from build123d import *

# Parameters (mm, degrees)
EXTRUDE1_DEPTH      = 8
EXTRUDE1_DEPTH_BACK = 8
SKETCH2_W           = 6.5
SKETCH2_H           = 12.5625
SKETCH3_W           = 94
SKETCH3_H           = 94
EXTRUDE2_DEPTH      = 31
SKETCH4_W           = 94
SKETCH4_H           = 47
EXTRUDE3_DEPTH      = 14
EXTRUDE3_DEPTH_BACK = 14
EXTRUDE4_DEPTH      = 2.06
EXTRUDE4_DEPTH_BACK = 2.06


with BuildPart() as part:
    # Sketch1 → Extrude1 (new body, two sides)
    with BuildSketch(Plane.XY) as extrude1_sk:
        with BuildLine():
            Line((-6.51, 14.5), (6.49, 14.5))
            ThreePointArc((6.49, 14.5), (10.317505243, 16.512584876), (14.256035557, 18.29815852))
            ThreePointArc((14.256035557, 18.29815852), (15.968337207, 18.822804929), (17.75042382, 19))
            Line((17.75042382, 19), (23.046668584, 19))
            ThreePointArc((23.046668584, 19), (24.290541726, 19.085889358), (25.51080482, 19.341927159))
            Line((25.51080482, 19.341927159), (35.534460964, 22.178335945))
            ThreePointArc((35.534460964, 22.178335945), (38.480369536, 24.039582758), (39.938965898, 27.204249197))
            Line((39.938965898, 27.204249197), (40.03902701, 27.893511518))
            ThreePointArc((40.03902701, 27.893511518), (39.384905735, 30.021406047), (37.324018346, 30.863161913))
            ThreePointArc((37.324018346, 30.863161913), (16.196447137, 28.065543342), (-4.25177913, 22.059631473))
            ThreePointArc((-4.25177913, 22.059631473), (-5.890644629, 20.775261015), (-6.51, 18.787325774))
            Line((-6.51, 18.787325774), (-6.51, 14.5))
        make_face()
    extrude(amount=EXTRUDE1_DEPTH)
    extrude(extrude1_sk.sketch, amount=-EXTRUDE1_DEPTH_BACK)

    # Sketch2 → Revolve1 (revolve)
    with BuildSketch(Plane.XY):
        with Locations((-3.26, 10.28125)):
            Rectangle(SKETCH2_W, SKETCH2_H)
    revolve(axis=Axis((-0.01, 16.5625, 0), (0, -1, 0)))

    # Sketch3 → Extrude2 (cut)
    with BuildSketch(Plane(origin=(0, 31, 0), x_dir=(-1, 0, 0), z_dir=(0, 1, 0))):
        with Locations((-7, -7)):
            Rectangle(SKETCH3_W, SKETCH3_H)
        with BuildLine():
            Line((-20.791020756, 4.081513031), (-36.5, 3.5))
            ThreePointArc((-36.5, 3.5), (-40, 0), (-36.5, -3.5))
            Line((-36.5, -3.5), (-20.791020756, -4.081513031))
            ThreePointArc((-20.791020756, -4.081513031), (-20.282143055, -4.074432197), (-19.7766212, -4.015658847))
            ThreePointArc((-19.7766212, -4.015658847), (-11.97399514, -3.733401658), (-4.362785826, -5.474130053))
            ThreePointArc((-4.362785826, -5.474130053), (7, 0), (-4.362785826, 5.474130053))
            ThreePointArc((-4.362785826, 5.474130053), (-11.97399514, 3.733401658), (-19.7766212, 4.015658847))
            ThreePointArc((-19.7766212, 4.015658847), (-20.282143055, 4.074432197), (-20.791020756, 4.081513031))
        make_face(mode=Mode.SUBTRACT)
    extrude(amount=-EXTRUDE2_DEPTH, mode=Mode.SUBTRACT)

    # Sketch4 → Extrude3 (cut, two sides)
    with BuildSketch(Plane.XY) as extrude3_sk:
        with Locations((7, 23.5)):
            Rectangle(SKETCH4_W, SKETCH4_H)
        with BuildLine():
            Line((-6.51, 18.787325774), (-6.51, 4.149977348))
            Line((-6.51, 4.149977348), (-6.360022652, 4))
            Line((-6.360022652, 4), (6.49, 4))
            Line((6.49, 4), (6.49, 9.643220966))
            ThreePointArc((6.49, 9.643220966), (7.726858035, 13.916382648), (11.05497769, 16.868220739))
            ThreePointArc((11.05497769, 16.868220739), (12.647037105, 17.602149488), (14.256035557, 18.29815852))
            ThreePointArc((14.256035557, 18.29815852), (15.968337207, 18.822804929), (17.75042382, 19))
            Line((17.75042382, 19), (23.046668584, 19))
            ThreePointArc((23.046668584, 19), (24.290541726, 19.085889358), (25.51080482, 19.341927159))
            Line((25.51080482, 19.341927159), (35.534460964, 22.178335945))
            ThreePointArc((35.534460964, 22.178335945), (38.480369536, 24.039582758), (39.938965898, 27.204249197))
            Line((39.938965898, 27.204249197), (40.03902701, 27.893511518))
            ThreePointArc((40.03902701, 27.893511518), (39.384905735, 30.021406047), (37.324018346, 30.863161913))
            ThreePointArc((37.324018346, 30.863161913), (16.196447137, 28.065543342), (-4.25177913, 22.059631473))
            ThreePointArc((-4.25177913, 22.059631473), (-5.890644629, 20.775261015), (-6.51, 18.787325774))
        make_face(mode=Mode.SUBTRACT)
    extrude(amount=EXTRUDE3_DEPTH, mode=Mode.SUBTRACT)
    extrude(extrude3_sk.sketch, amount=-EXTRUDE3_DEPTH_BACK, mode=Mode.SUBTRACT)

    # Sketch5 → Cut-Revolve1 (revolve, cut)
    with BuildSketch(Plane.XY):
        Polygon((0, 28.5), (4.926418831, 28.5), (4.3, 21.34), (4.3, 16), (2.5, 16), (2.5, 15), (4.15, 15), (4.15, 12.8), (5, 12.8), (5, 4.55), (5.25, 4.3), (5.25, 3), (0, 3), align=None)
    revolve(axis=Axis((0, 4, 0), (0, 1, 0)), mode=Mode.SUBTRACT)

    # Sketch6 → Revolve2 (revolve)
    with BuildSketch(Plane.XY):
        Polygon((0, 24.5), (4.3, 24.5), (4.3, 21.339), (2.5, 21.339), (2.5, 15), (4.15, 15), (4.15, 12.8), (5, 12.8), (5, 0.3), (4.7, 0), (0, 0), align=None)
    revolve(axis=Axis((0, 0, 0), (0, 1, 0)))

    # Sketch7 → Extrude4 (cut, two sides)
    with BuildSketch(Plane(origin=(0, 24.5, 0), x_dir=(-1, 0, 0), z_dir=(0, 1, 0))) as extrude4_sk:
        with BuildLine():
            ThreePointArc((1.903841526, -0.437854927), (2.25, 0), (1.903841526, 0.437854927))
            ThreePointArc((1.903841526, 0.437854927), (1.403569191, 0.81035105), (1.331114253, 1.429847663))
            ThreePointArc((1.331114253, 1.429847663), (1.125, 1.948557159), (0.572727273, 1.86770259))
            ThreePointArc((0.572727273, 1.86770259), (0, 1.620702101), (-0.572727273, 1.86770259))
            ThreePointArc((-0.572727273, 1.86770259), (-1.125, 1.948557159), (-1.331114253, 1.429847663))
            ThreePointArc((-1.331114253, 1.429847663), (-1.403569191, 0.81035105), (-1.903841526, 0.437854927))
            ThreePointArc((-1.903841526, 0.437854927), (-2.25, 0), (-1.903841526, -0.437854927))
            ThreePointArc((-1.903841526, -0.437854927), (-1.403569191, -0.81035105), (-1.331114253, -1.429847663))
            ThreePointArc((-1.331114253, -1.429847663), (-1.125, -1.948557159), (-0.572727273, -1.86770259))
            ThreePointArc((-0.572727273, -1.86770259), (0, -1.620702101), (0.572727273, -1.86770259))
            ThreePointArc((0.572727273, -1.86770259), (1.125, -1.948557159), (1.331114253, -1.429847663))
            ThreePointArc((1.331114253, -1.429847663), (1.403569191, -0.81035105), (1.903841526, -0.437854927))
        make_face()
    extrude(amount=EXTRUDE4_DEPTH, mode=Mode.SUBTRACT)
    extrude(extrude4_sk.sketch, amount=-EXTRUDE4_DEPTH_BACK, mode=Mode.SUBTRACT)

    # Sketch8 → Cut-Revolve2 (revolve, cut)
    with BuildSketch(Plane.XY):
        Polygon((0, 12.419415637), (2.4585, 11), (2.4585, 0.5415), (3, 0), (0, 0), align=None)
    revolve(axis=Axis((0, 0, 0), (0, 1, 0)), mode=Mode.SUBTRACT)


solid = part.part
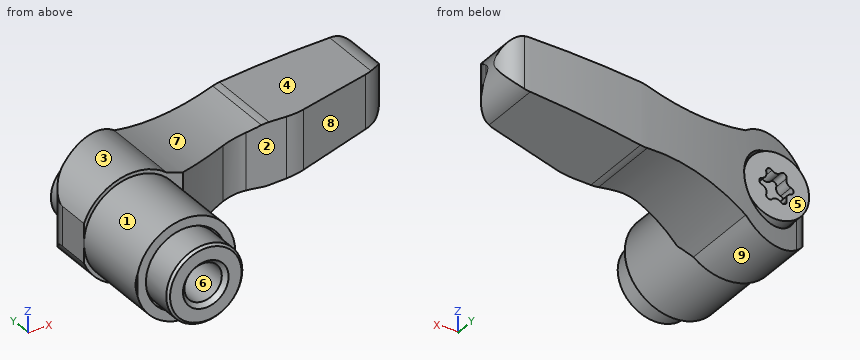
Verification items for the finished model (mm, model axes). Face numbers are marked on the shaded views. A direction names the side the tool comes from. Coordinates: 2 decimals unless noted, no trailing zeros. Order: outer loops, then holes, each group sorted by start corner. A loop starts at its lowest first (then second) coordinate and runs counter-clockwise, first axis right, second up. Notation, with made-up numbers: (-15, 81) -> (-2, 81) arc R19 cw to (-2, 114) -> close; hole circle Ø11 at (17, 70). An arc over 180 degrees is marked (long way). Put each result on its own line as item: value. Start each with the question number.
1. Cross-section at A-A, the plane y = 20.5. Record the boundary of the cut face in (x, z), then the cut area to 3 significant figures.
2. Cross-section at D-D, the plane x = 21.5. Record the boundary of the cut face in (y, z).
3. Cross-section at C-C, the plane y = 24. Count the separate pieces of the cut face and the enclosed holes in it, then the cut area to 3 significant figures.
4. Go/stop test with flat-tipped pins: pin 1 Ø3 at (y, z) = (14.5, -4.5) entering from +X; pin 2 Ø1 at (x, z) = (3, 0.5) entering from +Y; pin 3 Ø4 at (x, z) = (18, -2.5) entering from +Y. Record where each tip stops, or that it passes through.
5. Material ranges on L1, parallel to Z at x = 0, y = 19.65; L2, parallel to Z at x = 0, y = 8; L3, parallel to Y at x = 4, z = -0.5, recorded low to high. Write a range as [from, to].
6. Cross-section at B-B, the plane x = 6. Record the boundary of the cut face in (y, z).
7. Access from +Z, -Z, +X, -X, +Y, -Y to the whole of each face (thin tool, end or side, straight path). Record for the marked faces 1, 2, 3, 4 and 5.
8. Mould release check, pull along X, two halves, no side actions. Record for the marked faces 6, 7, 8 and 9: released by +X, released by -X, zero draft, split by the parting line, or undercut.
Computed:
1. outline: (-6.06, -3.5) arc R7 ccw to (4.36, -5.47) arc R30 cw to (19.78, -4.02) arc R5 ccw to (20.79, -4.08) -> (29.6, -3.76) -> (29.6, 3.76) -> (20.79, 4.08) arc R5 ccw to (19.78, 4.02) arc R30 cw to (4.36, 5.47) arc R7 ccw to (-6.06, 3.5) -> close; circle Ø5 at (0, 0); hole circle Ø8.6 at (0, 0)
1. area: 293 mm2
2. outline: (19, -4.06) -> (29.08, -4.06) -> (29.08, 4.06) -> (19, 4.06) -> close
3. separate pieces: 2
3. enclosed holes: 1
3. area: 331 mm2
4. pin 1: x = 9.2
4. pin 2: y = 24.5
4. pin 3: y = 28.82
5. L1: [-7, -4.3], [-2.5, 2.5], [4.3, 7]
5. L2: [-6.5, -2.46], [2.46, 6.5]
5. L3: [0, 16], [21.34, 24.5]
6. outline: (4, -2.48) -> (14.5, -2.48) -> (14.5, -4.92) -> (25.5, -4.92) -> (25.5, 4.92) -> (14.5, 4.92) -> (14.5, 2.48) -> (4, 2.48) -> close
7. face 1: -Y
7. face 2: +Z, -Z, +X, -Y
7. face 3: +Z, +Y, -Y
7. face 4: +Z, +X, +Y, -Y
7. face 5: -X, +Y
8. face 6: undercut
8. face 7: undercut
8. face 8: released by +X
8. face 9: split by the parting line
